Study the drawing (mm; zero at the part's minimum x, y, z) and answer. A direction names the side the tool comes from. Round coordinates to 2 decimals unless told otherwise and drop trailing zeros. Write each loop counter-clockwise with the first axis right and the second up, starting at its lowest first coordinate (ties: lowest second). Pieces come first, ordered by that corner, then holes.
(1) Each of these flat-tipped pins is pushed along its axis until it touches: pin 1 Ø5 at (y, z) = (24, 13.5) entering from -X; pin 2 Ø1 at (y, z) = (34, 10.5) entering from -X; pin 3 Ø5 at (x, z) = (26, 21) entering from -Y; pin 4 Ø9.5 at (y, z) = (20, 23.5) entering from +X. Where does it stop, or does it pass through?
(2) For the marked faces 1, 2 and 3, determine the directions among +Z, -Z, +X, -X, +Y, -Y from which every point of the face is accessible in a straight line to the end or side of a thin tool.
(3) Find the intervals of material crossed by probe 1 along X at (y, z) = (4.5, 9); probe 2 along Y at (x, z) = (22.5, 11); probe 3 along Y at (x, z) = (23.5, 25), in increasing order.
(4) A cutting plane is placed at A-A, the plane y = 6. Give the vertices of the cut face in (x, z).
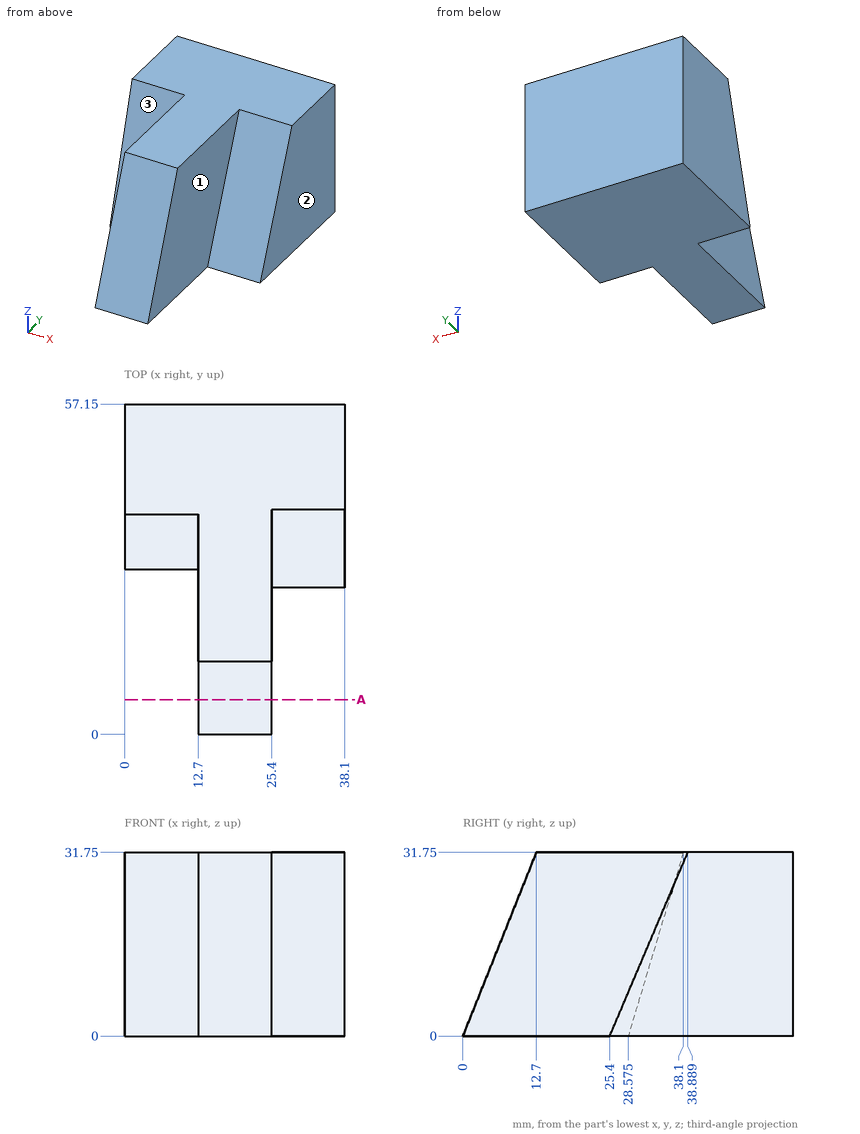
Solutions:
1. pin 1: stops at x = 12.7
1. pin 2: stops at x = 0
1. pin 3: stops at y = 7.43
1. pin 4: stops at x = 25.4
2. face 1: +Z, +X, -Y
2. face 2: +Z, -Z, +X, +Y, -Y
2. face 3: +Z, -X, -Y
3. probe 1: x = 12.7 to 25.4
3. probe 2: y = 4.4 to 57.15
3. probe 3: y = 10 to 57.15
4. outline: (12.7, 0) - (25.4, 0) - (25.4, 15) - (12.7, 15) - close
